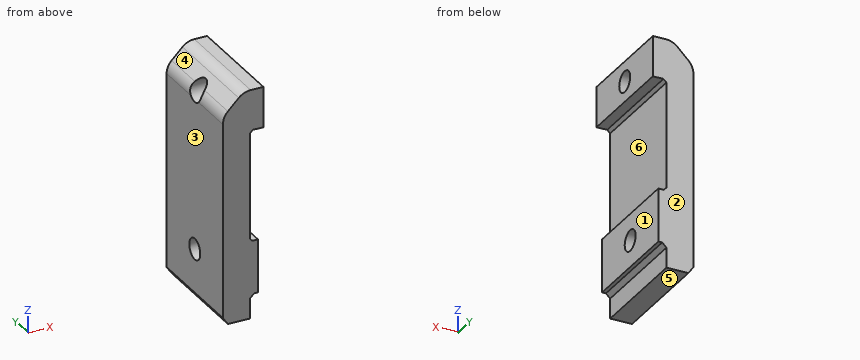
from build123d import *

# Parameters (mm, degrees)
EXTRUDE_1_DEPTH          = 16
CUT_EXTRUDE_1_DEPTH      = 31.882108434
CUT_EXTRUDE_1_DEPTH_BACK = 31.882108434
SKETCH_2_R               = 1.55


with BuildPart() as part:
    # ｽｹｯﾁ1 → ﾎﾞｽ - 押し出し1 (new body)
    with BuildSketch(Plane(origin=(0, 0, 0), x_dir=(1, 0, 0), z_dir=(0, 1, 0))):
        with BuildLine():
            Line((1.311036439, 22.922778474), (1.311036439, 25.896873144))
            Line((1.311036439, 25.896873144), (-1.944631198, 25.896873144))
            Line((-1.944631198, 25.896873144), (-2.690557808, 24.817055549))
            Line((-2.690557808, 24.817055549), (-2.676864245, 24.830749112))
            Line((-2.676864245, 24.830749112), (-2.676864245, 17.239005736))
            Line((-2.676864245, 17.239005736), (-2.676864245, -3.996970874))
            ThreePointArc((-2.676864245, -3.996970874), (-2.486563076, -4.953679455), (-1.944631198, -5.764737827))
            Line((-1.944631198, -5.764737827), (-0.338475216, -7.370893809))
            ThreePointArc((-0.338475216, -7.370893809), (0.472583156, -7.912825688), (1.429291737, -8.103126856))
            Line((1.429291737, -8.103126856), (3.323135755, -8.103126856))
            Line((3.323135755, -8.103126856), (3.323135755, -2.103126856))
            Line((3.323135755, -2.103126856), (1.751325003, -2.103126856))
            Line((1.751325003, -2.103126856), (1.311036439, -1.662838292))
            Line((1.311036439, -1.662838292), (1.311036439, 13.978392046))
            Line((1.311036439, 13.978392046), (1.674004174, 14.396873144))
            Line((1.674004174, 14.396873144), (2.511036439, 14.396873144))
            Line((2.511036439, 14.396873144), (2.511036439, 22.296873144))
            Line((2.511036439, 22.296873144), (1.936941769, 22.296873144))
            Line((1.936941769, 22.296873144), (1.311036439, 22.922778474))
        make_face()
    extrude(amount=EXTRUDE_1_DEPTH)

    # ｽｹｯﾁ2 → ｶｯﾄ - 押し出し1 (cut, two sides: drawn at the far end of the back side and taken through both)
    with BuildSketch(Plane(origin=(2.511036439, 0, 0), x_dir=(0, 0, -1), z_dir=(1, 0, 0)).offset(-CUT_EXTRUDE_1_DEPTH_BACK)):
        with Locations(Location((18.346873144, 8, 0), (0, 0, 180))):
            Circle(SKETCH_2_R)
        with Locations((-5.103126856, 8)):
            Circle(SKETCH_2_R)
    extrude(amount=CUT_EXTRUDE_1_DEPTH + CUT_EXTRUDE_1_DEPTH_BACK, mode=Mode.SUBTRACT)


solid = part.part
Input: part model. Units: mm. Frame: model coordinates. Face numbers are marked on the shaded views. A direction names the side the tool comes from. Give positions to 0.01 mm unless a question says otherwise; leave off trailing zeros. Write each loop counter-clockwise with the first axis right and the second up, starting at its lowest first coordinate (ties: lowest second). Pieces come first, ordered by that corner, then holes. Notation, with made-up numbers: M 33.25,-23.75 L 69.25,-23.75 A28 cw 69.25,-3.75 Z; hole C 5.5,34 d11. An arc over 180 degrees is marked long. Write item = value, one per line. Start each with the question number.
1) Cut plane A-A on y = 7.25. Count the separate pieces of the cut face and the enclosed holes in it, then the cut area to 3 significant figures.
2) Cut plane D-D on z = -15. Return the cut outline in (x, y), then the cut area to 3 significant figures.
3) First-contact query: pin 1 Ø1.5 at (y, z) = (13.5, 2) entering from -X; pin 2 Ø0.6 at (x, y) = (2.5, 9) entering from -Z; pin 3 Ø4.5 at (y, z) = (5.5, -8) entering from +X; pin 4 Ø5 at (y, z) = (8, 5.1) entering from +X. Flat tips, straight axial feed; report the tip coordinate or a pass-through.
4) Material intervals for line 1 along X through (y, z) = (13.75, -4); line 2 along Z through (x, y) = (2.75, 14); line 3 along Y through (x, z) = (0.25, -19), sorted ascending. Write a range as [from, to].
5) Draft query along Z for the marked faces 3, 4, 5 and 6. Return one class per face: +Z half, -Z half, draft (parallel to the pull), parting line (faces both ways), or undercut.
6) Reachability of the marked faces 1 and 2 from +Z, -Z, +X, -X, +Y, -Y: full face, straight path, thin tool, end or side. Return the list, or none.
7) Cut plane C-C on z = 0. Return the cut outline in (x, y), then the cut area to 3 significant figures.
Solved:
q1.separate_pieces = 3
q1.enclosed_holes = 0
q1.area = 123 mm2
q2.outline = M -2.68,0 L 2.51,0 L 2.51,16 L -2.68,16 Z
q2.area = 83.0 mm2
q3.pin_1 = -2.68
q3.pin_2 = -22.3
q3.pin_3 = 1.31
q3.pin_4 = 3.32
q4.line_1 = [-2.68, 1.31]
q4.line_2 = [2.1, 8.1]
q4.line_3 = [0, 6.59], [9.41, 16]
q5.face_3 = draft
q5.face_4 = +Z half
q5.face_5 = -Z half
q5.face_6 = undercut
q6.face_1 = -Z, +X, +Y, -Y
q6.face_2 = +Z, -Z, +X, -X, +Y
q7.outline = M -2.68,0 L 1.31,0 L 1.31,16 L -2.68,16 Z
q7.area = 63.8 mm2
